Autodesk Inventor part; units mm, degrees
sketch "Sketch1" plane through (0, 0, 0) normal (0, 0, 1) x (1, 0, 0)
  circle A0 centre (0, 0) radius 31.75
  circle A1 centre (0, 0) radius 3
  line L0 (0, -3) -> (0, 2.5) construction
  line L1 (0, 2.5) -> (1.6583, 2.5)
  line L2 (0, 2.5) -> (-1.6583, 2.5)
  dimension "d0" = 63.5
  dimension "d1" = 6
  dimension "d2" = 5.5
extrude "Extrusion1" add sketch "Sketch1" along normal blind 20.32 contours A0 | L1 L2 A1 picked at (-0.897, 2.6056)
sketch "Sketch2" plane through (0, 0, 0) normal (0, 1, 0) x (-1, 0, 0)
  line L0 (31.75, 7.62) -> (30.1625, 7.62)
  line L1 (30.1625, 7.62) -> (30.1625, 12.7)
  line L2 (30.1625, 12.7) -> (31.75, 12.7)
  line L3 (31.75, 7.62) -> (31.75, 12.7)
  line L4 (31.75, 0) -> (31.75, 7.62)
  line L5 (31.75, 20.32) -> (-31.75, 20.32)
  line L6 (31.75, 12.7) -> (31.75, 20.32)
  line L7 (0, -4.064) -> (0, 24.384)
  point P0 (0, 0)
  point P1 (31.75, 10.16)
  dimension "d5" = 5.08
  dimension "d6" = 1.5875
  dimension "d7" = 7.62
revolve "Revolution1" cut sketch "Sketch2" angle 360 about axis through (0, 0, -10) along (0, 0, 1)
The model under review builds one solid part; all positions refer to its coordinate system, in mm. A direction names the side the tool comes from. Coordinates: 2 decimals unless noted, no trailing zeros. Order: outer loops, then holes, each group sorted by start corner. A loop starts at its lowest first (then second) coordinate and runs counter-clockwise, first axis right, second up. Notation, with made-up numbers: (51, 50.5) -> (91, 50.5) arc R11 cw to (91, 71.5) -> close; hole circle Ø9 at (27, 78.5). An arc over 180 degrees is marked (long way). Answer in a Markdown table with one row per item.
(1) The part is to be moulded in two halves that separate along Z. For faces 1 (the flat face through (7, 0, 20.32)), 2 (the flat face through (-28, 12, 7.62)), 3 (the cylindrical face through (-6.883, 30.995, 3.757)), 4 (the flat face through (7, 0, 0)), say which applies: +Z half, -Z half, draft (parallel to the pull), parting line (faces both ways), or undercut.
Answers:
| item | result |
|---|---|
| face 1 | +Z half |
| face 2 | undercut |
| face 3 | draft |
| face 4 | -Z half |
(2) Machinability: for faces 5 (the flat face through (0, 2.5, 10)), 6 (the cylindrical face through (30.133, -1.326, 10.196)), which of the approach directions +Z, -Z, +X, -X, +Y, -Y give a long, thin tool a straight path to every point of the face, cutting with its end or side? Answer none if there is none.
Answers:
| item | result |
|---|---|
| face 5 | +Z, -Z |
| face 6 | none |
(3) Insertion check: pin 1 (1.5 mm diameter, centred on y = 21, z = 14.5, fed in from -X); pin 2 (2 mm diameter, centred on x = -2, z = 3.5, fed in from -Y); pin 3 (10 mm diameter, centred on x = -18, y = -9.5, fed in from -Z); pin 4 (5 mm diameter, centred on x = -2, z = 9, fed in from +Y). Each pin has a flat end and moves straight along its axis. Give the tip position at first contact, or say it passes through.
Answers:
| item | result |
|---|---|
| pin 1 | x = -24.45 |
| pin 2 | y = -31.73 |
| pin 3 | z = 0 |
| pin 4 | y = 31.75 |
(4) Wall thickness on line 1 along X through (y, z) = (0, 9.5); line 2 along Z through (x, y) = (23.5, 20.5); line 3 along Y through (x, z) = (0, 13.25): over which ranges is each line inside the solid? List them lowest first.
Answers:
| item | result |
|---|---|
| line 1 | -30.16 to -3, 3 to 30.16 |
| line 2 | 0 to 7.62, 12.7 to 20.32 |
| line 3 | -31.75 to -3, 2.5 to 31.75 |
(5) Consider section C-C (z = 17.25). Write out the cut boundary in (x, y).
Answers:
| item | result |
|---|---|
| outline | circle Ø63.5 at (0, 0); hole (-1.66, 2.5) arc R3 ccw (long way) to (1.66, 2.5) -> close |
(6) Consider section B-B (x = 0). Write out the cut boundary in (y, z).
Answers:
| item | result |
|---|---|
| outline | (-31.75, 0) -> (-3, 0) -> (-3, 20.32) -> (-31.75, 20.32) -> (-31.75, 12.7) -> (-30.16, 12.7) -> (-30.16, 7.62) -> (-31.75, 7.62) -> close; (2.5, 0) -> (31.75, 0) -> (31.75, 7.62) -> (30.16, 7.62) -> (30.16, 12.7) -> (31.75, 12.7) -> (31.75, 20.32) -> (2.5, 20.32) -> close |
(7) Consider section A-A (y = 0). Write out the cut boundary in (x, z).
Answers:
| item | result |
|---|---|
| outline | (-31.75, 0) -> (-3, 0) -> (-3, 20.32) -> (-31.75, 20.32) -> (-31.75, 12.7) -> (-30.16, 12.7) -> (-30.16, 7.62) -> (-31.75, 7.62) -> close; (3, 0) -> (31.75, 0) -> (31.75, 7.62) -> (30.16, 7.62) -> (30.16, 12.7) -> (31.75, 12.7) -> (31.75, 20.32) -> (3, 20.32) -> close |
(8) Consider section D-D (y = 12.5). Write out the cut boundary in (x, z).
Answers:
| item | result |
|---|---|
| outline | (-29.19, 0) -> (29.19, 0) -> (29.19, 7.62) -> (27.45, 7.62) -> (27.45, 12.7) -> (29.19, 12.7) -> (29.19, 20.32) -> (-29.19, 20.32) -> (-29.19, 12.7) -> (-27.45, 12.7) -> (-27.45, 7.62) -> (-29.19, 7.62) -> close |
